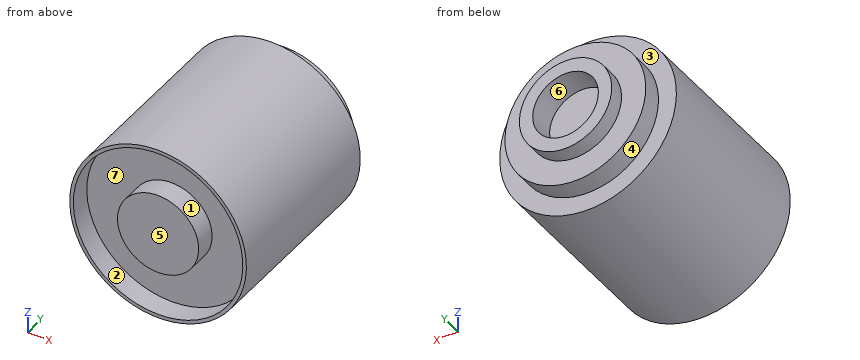
from build123d import *

# Parameters (mm, degrees)
SKETCH_5_R          = 37
EXTRUDE_1_DEPTH     = 76
EXTRUDE_2_REACH     = 101.389
SKETCH_4_R          = 29.5
EXTRUDE_3_REACH     = 107.015
SKETCH_1_R          = 19.34
SKETCH_2_R          = 13.75
CUT_EXTRUDE_1_DEPTH = 11.3
SKETCH_7_R          = 35.5
SKETCH_7_R_2        = 17
CUT_EXTRUDE_2_DEPTH = 9


with BuildPart() as part:
    # Эскиз5 → Бобышка-Вытянуть1 (new body)
    with BuildSketch(Plane(origin=(0, -15.05, 0), x_dir=(1, 0, 0), z_dir=(0, 1, 0))):
        with Locations(Location((0, 0, 0), (0, 0, 270))):
            Circle(SKETCH_5_R)
    extrude(amount=-EXTRUDE_1_DEPTH)

    # Эскиз4 → Бобышка-Вытянуть2 (add, up to next)
    with BuildSketch(Plane(origin=(0, -6.55, 0), x_dir=(1, 0, 0), z_dir=(0, 1, 0)), mode=Mode.PRIVATE) as extrude_2_sk1:
        with Locations(Location((0, 0, 0), (0, 0, 270))):
            Circle(SKETCH_4_R)
    extrude_2_tool1 = extrude(extrude_2_sk1.sketch, amount=-EXTRUDE_2_REACH, mode=Mode.PRIVATE) - part.part
    add(extrude_2_tool1.solids().sort_by_distance((0, -6.55, 0))[0])

    # Эскиз1 → Бобышка-Вытянуть3 (add, up to next)
    with BuildSketch(Plane(origin=(0, 0, 0), x_dir=(1, 0, 0), z_dir=(0, 1, 0)), mode=Mode.PRIVATE) as extrude_3_sk1:
        with Locations(Location((0, 0, 0), (0, 0, 270))):
            Circle(SKETCH_1_R)
    extrude_3_tool1 = extrude(extrude_3_sk1.sketch, amount=-EXTRUDE_3_REACH, mode=Mode.PRIVATE) - part.part
    add(extrude_3_tool1.solids().sort_by_distance((0, 0, 0))[0])

    # Эскиз2 → Вырез-Вытянуть1 (cut)
    with BuildSketch(Plane(origin=(0, -11.3, 0), x_dir=(1, 0, 0), z_dir=(0, 1, 0))):
        with Locations(Location((0, 0, 0), (0, 0, 270))):
            Circle(SKETCH_2_R)
    extrude(amount=CUT_EXTRUDE_1_DEPTH, mode=Mode.SUBTRACT)

    # Эскиз7 → Вырез-Вытянуть2 (cut)
    with BuildSketch(Plane.XZ.offset(91.05)):
        with Locations(Location((0, 0, 0), (0, 0, 270))):
            Circle(SKETCH_7_R)
        with Locations(Location((0, 0, 0), (0, 0, 270))):
            Circle(SKETCH_7_R_2, mode=Mode.SUBTRACT)
    extrude(amount=-CUT_EXTRUDE_2_DEPTH, mode=Mode.SUBTRACT)


solid = part.part
Check sheet for the modelled part. Datum: model origin and axes. Units: mm. Face numbers are marked on the shaded views. A direction names the side the tool comes from. Round coordinates to 2 decimals unless told otherwise and drop trailing zeros. Loops run counter-clockwise (first coordinate to the right, second up) from the corner with the lowest first, then second, coordinate; pieces in that order, holes last. Notation, with made-up numbers: M 82.25,21 L 89.25,21 A11 cw 89.25,35 Z; hole C -18,-12 d8. An arc over 180 degrees is marked long. One line per item, written item: value.
(1) Sectioned sample at D-D, the plane x = 15.5. Record the cut outline in (y, z).
Computed values:
outline: M -91.05,-33.6 L -15.05,-33.6 L -15.05,-25.1 L -6.55,-25.1 L -6.55,-11.57 L 0,-11.57 L 0,11.57 L -6.55,11.57 L -6.55,25.1 L -15.05,25.1 L -15.05,33.6 L -91.05,33.6 L -91.05,31.94 L -82.05,31.94 L -82.05,6.98 L -91.05,6.98 L -91.05,-6.98 L -82.05,-6.98 L -82.05,-31.94 L -91.05,-31.94 Z
(2) Sectioned sample at C-C, the plane y = -58.5. Record the cut outline in (x, z), then the cut area to 3 significant figures.
Computed values:
outline: C 0,0 d74
area: 4,300 mm^2
(3) Release check for a two-part mould opening along Z. For the marked faces 1, 2, 3 and 4 record: +Z half, -Z half, draft (parallel to the pull), parting line (faces both ways), or undercut.
Computed values:
face 1: undercut
face 2: undercut
face 3: draft
face 4: parting line
(4) Depth check by flat-ended pin: pin 1 Ø4 at (y, z) = (-64.5, -1) entering from -X; pin 2 Ø5 at (y, z) = (-19, 3) entering from +X; pin 3 Ø4 at (x, y) = (11.5, -37.5) entering from -Z. Enter the tip coordinate at first touch or a pass-through.
Computed values:
pin 1: stops at x = -37
pin 2: stops at x = 37
pin 3: stops at z = -35.76
(5) Sectioned sample at B-B, the plane x = 0. Record the cut outline in (y, z).
Computed values:
outline: M -91.05,-37 L -15.05,-37 L -15.05,-29.5 L -6.55,-29.5 L -6.55,-19.34 L 0,-19.34 L 0,-13.75 L -11.3,-13.75 L -11.3,13.75 L 0,13.75 L 0,19.34 L -6.55,19.34 L -6.55,29.5 L -15.05,29.5 L -15.05,37 L -91.05,37 L -91.05,35.5 L -82.05,35.5 L -82.05,17 L -91.05,17 L -91.05,-17 L -82.05,-17 L -82.05,-35.5 L -91.05,-35.5 Z
(6) Sectioned sample at A-A, the plane z = 0. Record the cut outline in (x, y), then the cut area to 3 significant figures.
Computed values:
outline: M -37,-91.05 L -35.5,-91.05 L -35.5,-82.05 L -17,-82.05 L -17,-91.05 L 17,-91.05 L 17,-82.05 L 35.5,-82.05 L 35.5,-91.05 L 37,-91.05 L 37,-15.05 L 29.5,-15.05 L 29.5,-6.55 L 19.34,-6.55 L 19.34,0 L 13.75,0 L 13.75,-11.3 L -13.75,-11.3 L -13.75,0 L -19.34,0 L -19.34,-6.55 L -29.5,-6.55 L -29.5,-15.05 L -37,-15.05 Z
area: 5,740 mm^2
(7) Thickness scan on line 1 (X direction, y = -86, z = 0); line 2 (X direction, y = -2, z = 0); line 3 (Y direction, x = -11, z = 7). Record the ranges inside material, lowest first.
Computed values:
line 1: x = -37 to -35.5, -17 to 17, 35.5 to 37
line 2: x = -19.34 to -13.75, 13.75 to 19.34
line 3: y = -91.05 to -11.3
(8) Access from +Z, -Z, +X, -X, +Y, -Y to the whole of each face (thin tool, end or side, straight path). Record for the marked faces 5, 6 and 7.
Computed values:
face 5: +Z, -Z, +X, -X, -Y
face 6: +Y
face 7: -Y
